Verification items for the finished model (mm, model axes). Face numbers are marked on the shaded views. A direction names the side the tool comes from. Give positions to 0.01 mm unless a question says otherwise; leave off trailing zeros. Loops run counter-clockwise (first coordinate to the right, second up) from the corner with the lowest first, then second, coordinate; pieces in that order, holes last. Notation, with made-up numbers: (51, 36.5) - (109, 36.5) arc R19 cw to (109, 73.5) - close; hole circle Ø3 at (11.25, 32.5). An arc over 180 degrees is marked (long way). One line per item, written item: value. Start each with the question number.
1. Sectioned sample at A-A (x = 42). Record the cut outline in (y, z), plus the area to 3 significant figures.
2. Sectioned sample at D-D (x = 77.5). Record the cut outline in (y, z).
3. Access from +Z, -Z, +X, -X, +Y, -Y to the whole of each face (thin tool, end or side, straight path). Record for the marked faces 5, 6 and 7.
4. Mould release check, pull along X, two halves, no side actions. Record for the marked faces 1, 2, 3 and 4: pulls with the +X half, pulls with the -X half, needs draft (parallel to the pull), parting line crosses it, or undercut.
5. Gauge pin test, flat ends, axial feed: pin 1 (12 mm diameter, centred on x = 8.5, y = 27, fed in from -Z); pin 2 (12.5 mm diameter, centred on y = 203.5, z = 24.5, fed in from -X); pin 3 (15.5 mm diameter, centred on x = 50.5, z = 31, fed in from -Y). Record the tip position at first contact, or that the pin passes through.
6. Scan lines: L1, parallel to X at y = 154, z = 20.5; L2, parallel to Z at x = 10, y = 86.5; L3, parallel to Y at x = 66.5, z = 29. Record each from-to range of solid material in increasing order. Write a range as [from, to].
7. Sectioned sample at B-B (y = 22). Record the cut outline in (x, z), plus the area to 3 significant figures.
8. Sectioned sample at C-C (z = -65). Record the cut outline in (x, y).
from build123d import *

# Parameters (mm, degrees)
EXTRUDE_1_DEPTH        = 41
EXTRUDE_2_DEPTH        = 10
SKETCH_3_R             = 11
CUT_EXTRUDE_1_DEPTH    = 10
SKETCH_4_W             = 83.5
SKETCH_4_H             = 41
EXTRUDE_3_DEPTH        = 250
CUT_EXTRUDE_2_DEPTH    = 309
EXTRUDE_5_DEPTH        = 83.5
EXTRUDE_6_DEPTH        = 41.75
FILLET_1_R             = 8
SKETCH_10_R            = 5.5
CUT_EXTRUDE_3_DEPTH    = 92
EXTRUDE_9_DEPTH        = 41.75
SKETCH_15_R            = 11
CUT_EXTRUDE_5_DEPTH    = 92.5
SKETCH_16_W            = 63.5
SKETCH_16_H            = 100
CUT_EXTRUDE_6_DEPTH    = 65
FILLET_3_R             = 30
CUT_EXTRUDE_7_DEPTH    = 37.75
SKETCH_19_W            = 70.175183739
SKETCH_19_H            = 41.669127314
CUT_EXTRUDE_8_DEPTH    = 90.5
HOLE_WIZARD_M5_1_D     = 4.2
HOLE_WIZARD_M5_1_DEPTH = 10
HOLE_WIZARD_M5_1_TIP   = 1.2618073
FILLET_5_R             = 10
CUT_EXTRUDE_9_DEPTH    = 31


with BuildPart() as part:
    # 草图1 → 凸台-拉伸1 (new body)
    with BuildSketch(Plane.XY):
        Polygon((0, 0), (0, 40), (83.5, 40), (83.5, 0), (73.5, 0), (73.5, 30), (10, 30), (10, 0), align=None)
    extrude(amount=EXTRUDE_1_DEPTH)

    # 草图2 → 凸台-拉伸2 (add)
    with BuildSketch(Plane(origin=(83.5, 0, 0), x_dir=(0, 0, -1), z_dir=(1, 0, 0))):
        with BuildLine():
            Line((-41, 0), (0, 0))
            ThreePointArc((0, 0), (-20.5, -20.5), (-41, 0))
        make_face()
    extrude_2 = extrude(amount=-EXTRUDE_2_DEPTH)

    # 草图3 → 切除-拉伸1 (cut)
    with BuildSketch(Plane(origin=(83.5, 0, 0), x_dir=(0, 0, -1), z_dir=(1, 0, 0))):
        with Locations(Location((-20.5, 0, 0), (0, 0, 90))):
            Circle(SKETCH_3_R)
    cut_extrude_1 = extrude(amount=-CUT_EXTRUDE_1_DEPTH, mode=Mode.SUBTRACT)

    # 镜向1: 凸台-拉伸2, 切除-拉伸1 across plane
    add(extrude_2.mirror(Plane(origin=(41.75, 0, 0), x_dir=(0, 0, 1), z_dir=(1, 0, 0))))
    add(cut_extrude_1.mirror(Plane(origin=(41.75, 0, 0), x_dir=(0, 0, 1), z_dir=(1, 0, 0))), mode=Mode.SUBTRACT)

    # 草图4 → 凸台-拉伸3 (add)
    with BuildSketch(Plane(origin=(0, 40, 0), x_dir=(1, 0, 0), z_dir=(0, 1, 0))):
        with Locations((41.75, -20.5)):
            Rectangle(SKETCH_4_W, SKETCH_4_H)
    extrude(amount=EXTRUDE_3_DEPTH)

    # 草图5 → 切除-拉伸2 (cut)
    with BuildSketch(Plane.XY.offset(41)):
        with BuildLine():
            Line((15, 45), (68.5, 45))
            ThreePointArc((68.5, 45), (72.035533906, 46.464466094), (73.5, 50))
            Line((73.5, 50), (73.5, 80))
            ThreePointArc((73.5, 80), (72.035533906, 83.535533906), (68.5, 85))
            Line((68.5, 85), (15, 85))
            ThreePointArc((15, 85), (11.464466094, 83.535533906), (10, 80))
            Line((10, 80), (10, 50))
            ThreePointArc((10, 50), (11.464466094, 46.464466094), (15, 45))
        make_face()
        with BuildLine():
            Line((10, 100), (10, 130))
            ThreePointArc((10, 130), (11.464466094, 133.535533906), (15, 135))
            Line((15, 135), (68.5, 135))
            ThreePointArc((68.5, 135), (72.035533906, 133.535533906), (73.5, 130))
            Line((73.5, 130), (73.5, 100))
            ThreePointArc((73.5, 100), (72.035533906, 96.464466094), (68.5, 95))
            Line((68.5, 95), (15, 95))
            ThreePointArc((15, 95), (11.464466094, 96.464466094), (10, 100))
        make_face()
        with BuildLine():
            Line((10, 150), (10, 180))
            ThreePointArc((10, 180), (11.464466094, 183.535533906), (15, 185))
            Line((15, 185), (68.5, 185))
            ThreePointArc((68.5, 185), (72.035533906, 183.535533906), (73.5, 180))
            Line((73.5, 180), (73.5, 150))
            ThreePointArc((73.5, 150), (72.035533906, 146.464466094), (68.5, 145))
            Line((68.5, 145), (15, 145))
            ThreePointArc((15, 145), (11.464466094, 146.464466094), (10, 150))
        make_face()
    extrude(amount=-CUT_EXTRUDE_2_DEPTH, mode=Mode.SUBTRACT)

    # 草图7 → 凸台-拉伸5 (add)
    with BuildSketch(Plane(origin=(83.5, 0, 0), x_dir=(0, 0, -1), z_dir=(1, 0, 0))):
        Polygon((0, 262.345150809), (112.486411563, 307.792611131), (97.127541233, 345.807149168), (-41, 290), align=None)
    extrude(amount=-EXTRUDE_5_DEPTH)

    # 草图8 → 凸台-拉伸6 (add, symmetric)
    with BuildSketch(Plane(origin=(41.75, 0, 0), x_dir=(0, 0, -1), z_dir=(1, 0, 0))):
        Polygon((0, 232.345150809), (0, 192.345150809), (55, 192.345150809), (55, 210.345150809), align=None)
    extrude(amount=EXTRUDE_6_DEPTH, both=True)

    # 圆角1
    fillet_1_edges = [part.edges().sort_by_distance(p)[0] for p in [
        (41.75, 192.345150809, -55),
    ]]
    fillet(fillet_1_edges, radius=FILLET_1_R)

    # 草图10 → 切除-拉伸3 (cut)
    with BuildSketch(Plane(origin=(83.5, 0, 0), x_dir=(0, 0, -1), z_dir=(1, 0, 0))):
        with Locations(Location((47, 200.345150809, 0), (0, 0, 90))):
            Circle(SKETCH_10_R)
    extrude(amount=-CUT_EXTRUDE_3_DEPTH, mode=Mode.SUBTRACT)

    # 草图14 → 凸台-拉伸9 (add, symmetric)
    with BuildSketch(Plane(origin=(41.75, 0, 0), x_dir=(0, 0, -1), z_dir=(1, 0, 0))):
        with BuildLine():
            Line((97.127541233, 345.807149168), (112.486411563, 307.792611131))
            ThreePointArc((112.486411563, 307.792611131), (123.814245417, 334.479315315), (97.127541233, 345.807149168))
        make_face()
    extrude(amount=EXTRUDE_9_DEPTH, both=True)

    # 草图15 → 切除-拉伸5 (cut, symmetric)
    with BuildSketch(Plane(origin=(83.5, 0, 0), x_dir=(0, 0, -1), z_dir=(1, 0, 0))):
        with Locations((104.806976398, 326.79988015)):
            Circle(SKETCH_15_R)
        with Locations((58.44778367, 308.069550479)):
            Circle(SKETCH_15_R)
    extrude(amount=CUT_EXTRUDE_5_DEPTH, both=True, mode=Mode.SUBTRACT)

    # 草图16 → 切除-拉伸6 (cut)
    with BuildSketch(Plane(origin=(0, 263.544767644, 106.47899781), x_dir=(1, 0, 0), z_dir=(0, 0.9271838545667882, 0.37460659341591007))):
        with Locations((41.75, 190.096726194)):
            Rectangle(SKETCH_16_W, SKETCH_16_H)
    extrude(amount=-CUT_EXTRUDE_6_DEPTH, mode=Mode.SUBTRACT)

    # 圆角3
    fillet_3_edges = [part.edges().sort_by_distance(p)[0] for p in [
        (41.75, 262.345150809, 0),
        (41.75, 290, 41),
    ]]
    fillet(fillet_3_edges, radius=FILLET_3_R)

    # 草图8<2> → 切除-拉伸7 (cut, symmetric)
    with BuildSketch(Plane(origin=(41.75, 0, 0), x_dir=(0, 0, -1), z_dir=(1, 0, 0))):
        Polygon((0, 232.345150809), (0, 192.345150809), (55, 192.345150809), (55, 210.345150809), align=None)
    extrude(amount=CUT_EXTRUDE_7_DEPTH, both=True, mode=Mode.SUBTRACT)

    # 草图19 → 切除-拉伸8 (cut)
    with BuildSketch(Plane(origin=(83.5, 0, 0), x_dir=(0, 0, -1), z_dir=(1, 0, 0))):
        with Locations((35.08759187, 211.510587152)):
            Rectangle(SKETCH_19_W, SKETCH_19_H)
    extrude(amount=-CUT_EXTRUDE_8_DEPTH, mode=Mode.SUBTRACT)

    # M5 螺纹孔的螺纹孔钻头1
    with Locations(Plane(origin=(66.75, 214, 0), x_dir=(-1, 0, 0), z_dir=(0, 0, -1))):
        with Locations((0, 0), (50, 0), (50, -20), (0, -20)):
            Hole(HOLE_WIZARD_M5_1_D / 2, depth=HOLE_WIZARD_M5_1_DEPTH)
            with Locations((0, 0, -(HOLE_WIZARD_M5_1_DEPTH + HOLE_WIZARD_M5_1_TIP / 2))):  # 118° drill point
                Cone(0, HOLE_WIZARD_M5_1_D / 2, HOLE_WIZARD_M5_1_TIP, mode=Mode.SUBTRACT)

    # 圆角5
    fillet_5_edges = [part.edges().sort_by_distance(p)[0] for p in [
        (10, 297.018655973, -31.09585996),
        (73.5, 297.018655973, -31.09585996),
    ]]
    fillet(fillet_5_edges, radius=FILLET_5_R)

    # 草图22 → 切除-拉伸9 (cut)
    with BuildSketch(Plane.XY.offset(41)):
        with BuildLine():
            Line((10, 190), (10, 230))
            ThreePointArc((10, 230), (11.464466094, 233.535533906), (15, 235))
            Line((15, 235), (68.5, 235))
            ThreePointArc((68.5, 235), (72.035533906, 233.535533906), (73.5, 230))
            Line((73.5, 230), (73.5, 190))
            Line((73.5, 190), (73.5, 177.902541229))
            Line((73.5, 177.902541229), (10, 177.902541229))
            Line((10, 177.902541229), (10, 190))
        make_face()
    extrude(amount=-CUT_EXTRUDE_9_DEPTH, mode=Mode.SUBTRACT)


solid = part.part
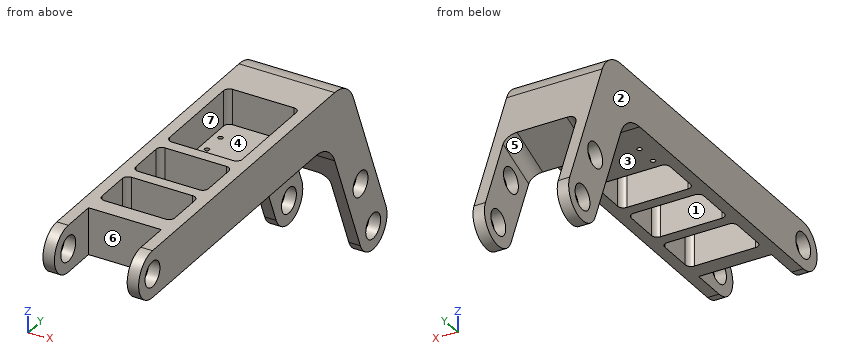
Results are:
1. outline: (30, 0) - (45, 0) - (45, 41) - (30, 41) - close; (85, 0) - (95, 0) - (95, 41) - (85, 41) - close; (135, 0) - (145, 0) - (145, 41) - (135, 41) - close; (185, 0) - (242.11, 0) arc R30 cw to (269.93, -18.76) - (278.01, -38.78) - (316.03, -23.42) - (297.58, 22.24) arc R30 ccw to (269.76, 41) - (235, 41) - (235, 10) - (185, 10) - close
1. area: 5,900 mm^2
2. outline: (0, 0) - (242.11, 0) arc R30 cw to (269.93, -18.76) - (307.79, -112.49) arc R20.5 ccw to (345.81, -97.13) - (297.58, 22.24) arc R30 ccw to (269.76, 41) - (0, 41) arc R20.5 ccw to start; hole circle Ø22 at (0, 20.5); hole circle Ø22 at (308.07, -58.45); hole circle Ø22 at (326.8, -104.81)
3. face 5: -Z, +Y
3. face 6: +Z, -Z, -Y
3. face 7: +Z
4. face 1: undercut
4. face 2: pulls with the -X half
4. face 3: needs draft
4. face 4: undercut
5. pin 1: stops at z = 0
5. pin 2: stops at x = 0
5. pin 3: stops at y = 30
6. L1: x = [0, 10], [73.5, 83.5]
6. L2: z = [0, 41]
6. L3: y = [30, 45], [85, 95], [135, 145], [235, 293.76]
7. outline: (0, 0) - (10, 0) - (10, 41) - (0, 41) - close; (73.5, 0) - (83.5, 0) - (83.5, 41) - (73.5, 41) - close
7. area: 820 mm^2
8. outline: (0, 288.61) - (10, 288.61) - (10, 299.23) - (0, 299.23) - close; (0, 316.91) - (10, 316.91) - (10, 332.83) - (0, 332.83) - close; (73.5, 288.61) - (83.5, 288.61) - (83.5, 299.23) - (73.5, 299.23) - close; (73.5, 316.91) - (83.5, 316.91) - (83.5, 332.83) - (73.5, 332.83) - close
